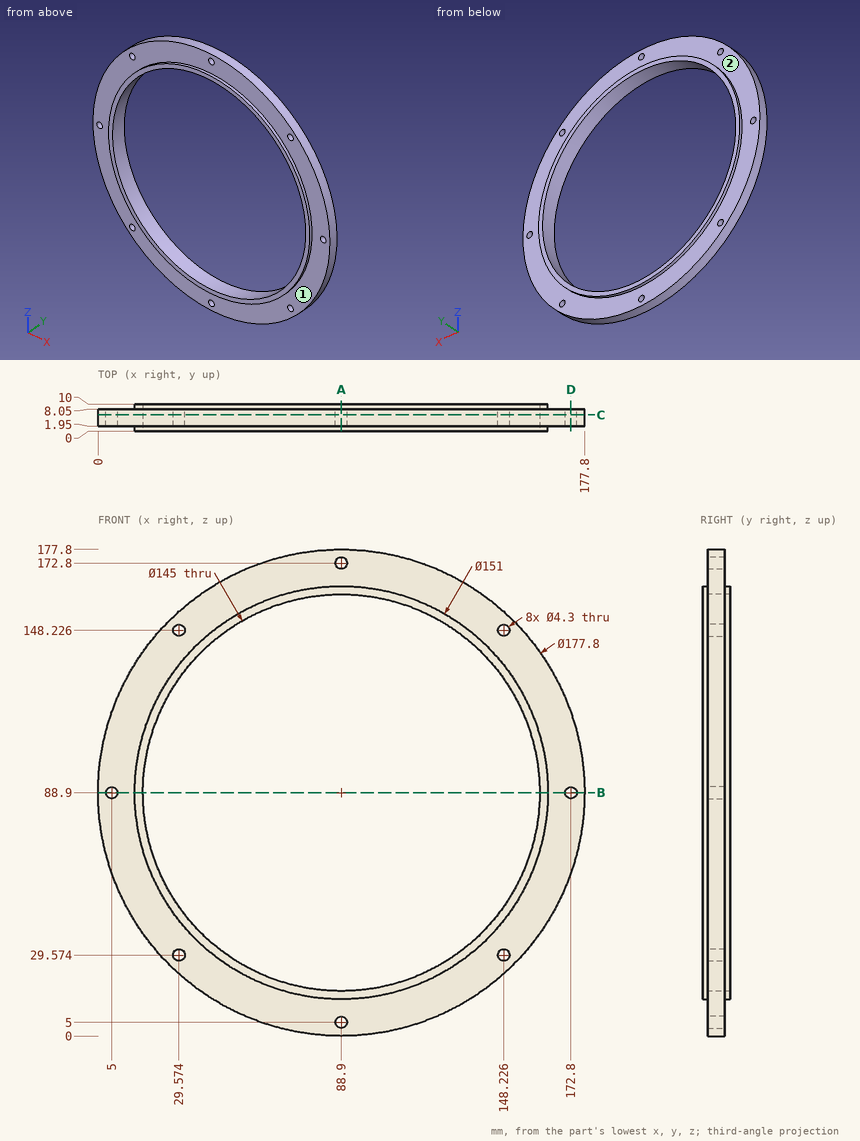
Print and shaded views of the part. All mm, measured from the part's lowest x, y and z. A direction names the side the tool comes from. Round coordinates to 2 decimals unless told otherwise and drop trailing zeros. Write each loop counter-clockwise with the first axis right and the second up, starting at its lowest first coordinate (ties: lowest second). Pieces come first, ordered by that corner, then holes. Notation, with made-up numbers: (19, 83) - (24, 83) arc R8 ccw to (24, 91) - close; hole circle Ø5 at (59, -10.75). An arc over 180 degrees is marked (long way). One line per item, written item: value.
(1) Drop flat-ended pins along their axis: P1, Ø6, axis at x = 29, y = 6, coming from the -Z side (1 decimal); P2, Ø6, axis at y = 2.5, z = 69, coming from the -X side; P3, Ø5, axis at x = 148.23, z = 148.23, coming from the -Y side; P4, Ø4, axis at x = 29.57, z = 148.23, coming from the +Y side (3 decimals). Give the stop position or say it passes through.
Values follow:
P1: stops at z = 20.6
P2: stops at x = 1.62
P3: stops at y = 1.95
P4: passes through
(2) 3-axis set-ups, long thin cutter, end or side, ignore diameter. For the marked faces 1 and 2: which of +Z, -Z, +X, -X, +Y, -Y reach the whole face in a straight line?
Values follow:
face 1: -Y
face 2: +Y
(3) Cut at B-B, the plane z = 88.9. Give the cut face in (x, y), plus the area to 3 significant figures.
Values follow:
outline: (0, 1.95) - (2.85, 1.95) - (2.85, 8.05) - (0, 8.05) - close; (7.15, 1.95) - (13.4, 1.95) - (13.4, 0) - (16.4, 0) - (16.4, 10) - (13.4, 10) - (13.4, 8.05) - (7.15, 8.05) - close; (161.4, 0) - (164.4, 0) - (164.4, 1.95) - (170.65, 1.95) - (170.65, 8.05) - (164.4, 8.05) - (164.4, 10) - (161.4, 10) - close; (174.95, 1.95) - (177.8, 1.95) - (177.8, 8.05) - (174.95, 8.05) - close
area: 171 mm²
(4) Cut at C-C, the plane y = 6. Give the number of separate pieces and of enclosed holes in the cut face, plus the area to 3 significant figures.
Values follow:
separate pieces: 1
enclosed holes: 9
area: 8,200 mm²
(5) Wall check: probe 1 along X at (y, z) = (3.25, 88.9); probe 2 along Z at (x, y) = (90, 6); probe 3 along Y at (x, z) = (140.5, 26). Give the ranges that are in metal, low to high.
Values follow:
probe 1: x = 0 to 2.85, 7.15 to 16.4, 161.4 to 170.65, 174.95 to 177.8
probe 2: z = 0.01 to 3.15, 6.85 to 16.41, 161.39 to 170.95, 174.65 to 177.79
probe 3: y = 1.95 to 8.05
(6) Cut at A-A, the plane x = 88.9. Give the cut face in (y, z).
Values follow:
outline: (0, 13.4) - (1.95, 13.4) - (1.95, 7.15) - (8.05, 7.15) - (8.05, 13.4) - (10, 13.4) - (10, 16.4) - (0, 16.4) - close; (0, 161.4) - (10, 161.4) - (10, 164.4) - (8.05, 164.4) - (8.05, 170.65) - (1.95, 170.65) - (1.95, 164.4) - (0, 164.4) - close; (1.95, 0) - (8.05, 0) - (8.05, 2.85) - (1.95, 2.85) - close; (1.95, 174.95) - (8.05, 174.95) - (8.05, 177.8) - (1.95, 177.8) - close
(7) Cut at D-D, the plane x = 172.8. Give the cut face in (y, z), plus the area to 3 significant figures.
Values follow:
outline: (1.95, 59.51) - (8.05, 59.51) - (8.05, 86.75) - (1.95, 86.75) - close; (1.95, 91.05) - (8.05, 91.05) - (8.05, 118.29) - (1.95, 118.29) - close
area: 332 mm²
